from build123d import *

# Parameters (mm, degrees)
F0_W     = 70
F0_H     = 60
F1_DEPTH = 20
F2_R     = 7
F3_T     = -3
F4_R     = 4.7885075057
F4_R_2   = 3.7026235456
F5_DEPTH = 1


with BuildPart() as f1:
    # F0 (on Front) → F1 (new body)
    with BuildSketch(Plane.XZ):
        Rectangle(F0_W, F0_H)
    extrude(amount=F1_DEPTH)

    # F2
    f2_edges = [f1.edges().sort_by_distance(p)[0] for p in [
        (35, -10, -30),
        (-35, -10, -30),
        (35, -10, 30),
        (-35, -10, 30),
    ]]
    fillet(f2_edges, radius=F2_R)

    # F3
    f3_openings = [f1.faces().sort_by_distance(p)[0] for p in [
        (0, 0, 0),
    ]]
    offset(amount=F3_T, openings=f3_openings)

    # F4 (on face) → F5 (cut)
    with BuildSketch(Plane.XZ.offset(20)):
        with BuildLine():
            ThreePointArc((5.9756954083, -21.3208798361), (7.5060376285, -18.8306109679), (8.0398977368, -15.9568712908))
            ThreePointArc((8.0398977368, -15.9568712908), (7.9036150749, -14.4863732956), (7.4994094473, -13.0659666184))
            Line((7.4994094473, -13.0659666184), (6.1305917901, -14.4159711191))
            ThreePointArc((6.1305917901, -14.4159711191), (6.2842749217, -15.2041179655), (6.3357852508, -16.0054547502))
            ThreePointArc((6.3357852508, -16.0054547502), (-5.5540754685, -18.7377869694), (3.9501702088, -11.0890131208))
            Line((3.9501702088, -11.0890131208), (5.196705387, -9.840010404))
            ThreePointArc((5.196705387, -9.840010404), (-7.9557042611, -15.6118703464), (4.6505361801, -22.4953976897))
            ThreePointArc((4.6505361801, -22.4953976897), (5.3457061154, -21.9449090553), (5.9756954083, -21.3208798361))
        make_face()
        with BuildLine():
            Line((0.0383761635, -19.0379637991), (5.7637177193, -13.3913118671))
            ThreePointArc((5.7637177193, -13.3913118671), (5.3063853455, -12.5665425426), (4.7303228045, -11.8198503118))
            Line((4.7303228045, -11.8198503118), (0.0383761635, -16.4483864674))
            Line((0.0383761635, -16.4483864674), (-2.3087403007, -14.0691147408))
            ThreePointArc((-2.3087403007, -14.0691147408), (-3.6156147651, -14.0808212911), (-3.5627264086, -15.386677612))
            Line((-3.5627264086, -15.386677612), (0.0383761635, -19.0379637991))
        make_face()
        with BuildLine():
            Line((5.7637177193, -13.3913118671), (7.0574382874, -12.1153723141))
            ThreePointArc((7.0574382874, -12.1153723141), (6.5608204438, -11.3219960932), (5.9749529426, -10.5920410388))
            Line((5.9749529426, -10.5920410388), (4.7303228045, -11.8198503118))
            ThreePointArc((4.7303228045, -11.8198503118), (5.3063853455, -12.5665425426), (5.7637177193, -13.3913118671))
        make_face()
        with BuildLine():
            ThreePointArc((5.9749529426, -10.5920410388), (6.5608204438, -11.3219960932), (7.0574382874, -12.1153723141))
            Line((7.0574382874, -12.1153723141), (10.3152280376, -8.9023579275))
            ThreePointArc((10.3152280376, -8.9023579275), (10.3242561937, -7.5976353085), (9.0195335747, -7.5886071525))
            Line((9.0195335747, -7.5886071525), (5.9749529426, -10.5920410388))
        make_face()
        with BuildLine():
            Line((-25.463836038, 14.5788419077), (-29.0132504877, 14.5788419077))
            Line((-29.0132504877, 14.5788419077), (-29.0132504877, 5.0767470373))
            Line((-29.0132504877, 5.0767470373), (-24.9086179807, 5.0767470373))
            ThreePointArc((-24.9086179807, 5.0767470373), (-22.7022924412, 7.5970867281), (-24.2285804935, 10.5787690258))
            ThreePointArc((-24.2285804935, 10.5787690258), (-23.7062839611, 12.9308235072), (-25.463836038, 14.5788419077))
        make_face()
        with BuildLine():
            Line((-27.9734000776, 10.8749483858), (-27.9734000776, 13.5894283968))
            Line((-27.9734000776, 13.5894283968), (-25.6162118383, 13.5894283968))
            ThreePointArc((-25.6162118383, 13.5894283968), (-24.6244842165, 12.2231458353), (-25.6406610471, 10.8749483858))
            Line((-25.6406610471, 10.8749483858), (-27.9734000776, 10.8749483858))
        make_face(mode=Mode.SUBTRACT)
        with BuildLine():
            Line((-27.9640843056, 9.8444300713), (-25.0821946304, 9.8444300713))
            ThreePointArc((-25.0821946304, 9.8444300713), (-23.7118512956, 8.0211258), (-25.0821946304, 6.1978215287))
            Line((-25.0821946304, 6.1978215287), (-27.9640843056, 6.188870993))
            Line((-27.9640843056, 6.188870993), (-27.9640843056, 9.8444300713))
        make_face(mode=Mode.SUBTRACT)
        with BuildLine():
            ThreePointArc((-19.3660976033, 14.2887552617), (-19.8752782584, 14.8065162395), (-20.40147499, 14.30605808))
            Line((-20.40147499, 14.30605808), (-20.40147499, 5.4078511567))
            ThreePointArc((-20.40147499, 5.4078511567), (-19.884282799, 5.1317819915), (-19.3660976033, 5.405982738))
            Line((-19.3660976033, 5.405982738), (-19.3660976033, 14.2887552617))
        make_face()
        with Locations((-12.3437182241, 9.891309084)):
            Circle(F4_R)
        with Locations((-12.3052396193, 9.8635797819)):
            Circle(F4_R_2, mode=Mode.SUBTRACT)
        Polygon((0.060495557, 14.6499899539), (-6.2339946938, 14.6499899539), (-6.2279876776, 13.6288518889), (-3.5691043968, 13.6288518889), (-3.5691043968, 5.3356449452), (-2.5498712742, 5.3356449452), (-2.5498712742, 13.6288518889), (0.060495557, 13.6288518889), align=None)
        with BuildLine():
            ThreePointArc((0.060495557, 13.6288518889), (0.5710645895, 14.1394209214), (0.060495557, 14.6499899539))
            Line((0.060495557, 14.6499899539), (0.060495557, 13.6288518889))
        make_face()
        with BuildLine():
            Line((-6.2279876776, 13.6288518889), (-6.2339946938, 14.6499899539))
            ThreePointArc((-6.2339946938, 14.6499899539), (-6.7385655444, 14.13643503), (-6.2279876776, 13.6288518889))
        make_face()
        with BuildLine():
            Line((5.68894728, 14.6499899539), (2.3992179348, 14.6499899539))
            Line((2.3992179348, 14.6499899539), (2.3992179348, 5.4546332436))
            ThreePointArc((2.3992179348, 5.4546332436), (2.9464930191, 5.1446017563), (3.4937681035, 5.4546332436))
            Line((3.4937681035, 5.4546332436), (3.4937681035, 8.8353623544))
            Line((3.4937681035, 8.8353623544), (5.4684750956, 8.8353623544))
            Line((5.4684750956, 8.8353623544), (7.6643496496, 5.2591634276))
            ThreePointArc((7.6643496496, 5.2591634276), (8.3467179976, 5.2108037756), (8.6122971182, 5.8412266091))
            Line((8.6122971182, 5.8412266091), (6.5826675849, 9.1466790748))
            ThreePointArc((6.5826675849, 9.1466790748), (8.1293427353, 12.2220783511), (5.68894728, 14.6499899539))
        make_face()
        with BuildLine():
            ThreePointArc((5.68894728, 13.6319459919), (7.0831009819, 11.7494924749), (5.5949211536, 9.9404549997))
            Line((5.5949211536, 9.9404549997), (3.3746365671, 9.9404549997))
            Line((3.3746365671, 9.9404549997), (3.3746365671, 13.6319459919))
            Line((3.3746365671, 13.6319459919), (5.68894728, 13.6319459919))
        make_face(mode=Mode.SUBTRACT)
        with BuildLine():
            ThreePointArc((14.7096056189, 14.4168665306), (14.3134062852, 14.6801129854), (13.9264534318, 14.4034541752))
            Line((13.9264534318, 14.4034541752), (10.6487381189, 5.9825136642))
            ThreePointArc((10.6487381189, 5.9825136642), (10.9675570687, 5.2573357806), (11.6927349523, 5.5761547304))
            Line((11.6927349523, 5.5761547304), (12.7655428348, 8.3323585177))
            Line((12.7655428348, 8.3323585177), (16.0099739306, 8.3323585177))
            Line((16.0099739306, 8.3323585177), (17.1330149852, 5.5268825081))
            ThreePointArc((17.1330149852, 5.5268825081), (17.8181026735, 5.2334854183), (18.1114997633, 5.9185731066))
            Line((18.1114997633, 5.9185731066), (14.7096056189, 14.4168665306))
        make_face()
        Polygon((13.1405137187, 9.48174586), (14.4126430381, 12.6535973069), (15.6418385154, 9.48174586), align=None, mode=Mode.SUBTRACT)
        with BuildLine():
            ThreePointArc((27.6586074546, 10.8364686124), (27.7543057203, 10.3589358747), (27.7863908123, 9.8729665129))
            ThreePointArc((27.7863908123, 9.8729665129), (20.7773970324, 8.2330148821), (26.3312045231, 12.8123879303))
            Line((26.3312045231, 12.8123879303), (27.0641849046, 13.6325057938))
            ThreePointArc((27.0641849046, 13.6325057938), (19.2418374627, 10.0479724553), (26.81568619, 5.9644918061))
            ThreePointArc((26.81568619, 5.9644918061), (27.2455005085, 6.3059753785), (27.6335724386, 6.6942427552))
            ThreePointArc((27.6335724386, 6.6942427552), (28.5370532464, 8.1811527366), (28.851969289, 9.8922946796))
            ThreePointArc((28.851969289, 9.8922946796), (28.7631907726, 10.8118138528), (28.5001349107, 11.6973638223))
            Line((28.5001349107, 11.6973638223), (27.6586074546, 10.8364686124))
        make_face()
        with BuildLine():
            Line((24.0681641205, 8.0956717688), (27.4159314963, 11.4858697823))
            ThreePointArc((27.4159314963, 11.4858697823), (27.1680184196, 11.9196861576), (26.8638629672, 12.316103869))
            Line((26.8638629672, 12.316103869), (24.0900374708, 9.5071220515))
            Line((24.0900374708, 9.5071220515), (22.775273925, 10.8054304358))
            ThreePointArc((22.775273925, 10.8054304358), (22.0626570945, 10.8039400184), (22.0641475119, 10.0913231879))
            Line((22.0641475119, 10.0913231879), (24.0681641205, 8.0956717688))
        make_face()
        with BuildLine():
            ThreePointArc((27.6335724386, 6.6942427552), (27.2455005085, 6.3059753785), (26.81568619, 5.9644918061))
            Line((26.81568619, 5.9644918061), (28.4407067429, 4.1904454021))
            ThreePointArc((28.4407067429, 4.1904454021), (29.214969102, 4.1564992903), (29.2489152138, 4.9307616493))
            Line((29.2489152138, 4.9307616493), (27.6335724386, 6.6942427552))
        make_face()
        with BuildLine():
            ThreePointArc((27.6311249444, 13.0930903614), (27.9416464389, 12.7068871234), (28.2107508353, 12.2907629071))
            Line((28.2107508353, 12.2907629071), (29.647856175, 13.7460825638))
            ThreePointArc((29.647856175, 13.7460825638), (29.6435095117, 14.4363306609), (28.9532614146, 14.4319839976))
            Line((28.9532614146, 14.4319839976), (27.6311249444, 13.0930903614))
        make_face()
        with BuildLine():
            ThreePointArc((26.8638629672, 12.316103869), (27.1680184196, 11.9196861576), (27.4159314963, 11.4858697823))
            Line((27.4159314963, 11.4858697823), (28.2107508353, 12.2907629071))
            ThreePointArc((28.2107508353, 12.2907629071), (27.9416464389, 12.7068871234), (27.6311249444, 13.0930903614))
            Line((27.6311249444, 13.0930903614), (26.8638629672, 12.316103869))
        make_face()
    extrude(amount=-F5_DEPTH, mode=Mode.SUBTRACT)


solid = f1.part
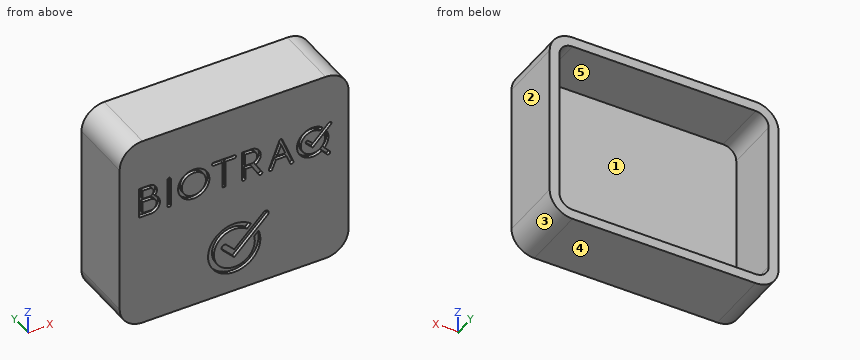
Source: CAD feature listing. Evaluate the final solid. Frame: model axes, mm. Face numbers are marked on the shaded views. A direction names the side the tool comes from. Round coordinates to 2 decimals unless told otherwise and drop trailing zeros. Loops run counter-clockwise (first coordinate to the right, second up) from the corner with the lowest first, then second, coordinate; pieces in that order, holes last.
Q1. Ray query, line 1 (X direction, y = -6.5, z = 17); line 2 (Z direction, x = -8, y = -10.5); line 3 (Y direction, x = -15, z = -20). Return the intervals inside material, ascending.
Q2. First-contact query: P1, Ø8.5, axis at x = -12.34, z = 9.89, coming from the +Y side. Flat tip, straight axial feed; report the tip coordinate or a pass-through.
Q3. Section A-A, the plane y = -13.75. Return loops of the section in (x, z).
Q4. Section D-D, the plane x = -12.5. Return loops of the section in (y, z).
Q5. Access query for the marked faces 1 and 2. Directions: +Z, -Z, +X, -X, +Y, -Y. A direction counts if a zero-diameter tool reaches every point of the face in a straight line with its end or side. Return the directions, or none.
Q6. Mould query, pull axis X, two halves, no side actions, for the marked faces 3, 4 and 5. Classes: pulls with the +X half, pulls with the -X half, needs draft (parallel to the pull), parting line crosses it, or undercut.
Q7. Section B-B, the plane z = 18. Return loops of the section in (x, y), plus the area to 3 significant figures.
Q8. Section C-C, the plane x = -26.5. Return loops of the section in (y, z), plus the area to 3 significant figures.
Solutions:
1. line 1: x = -35 to -32, 32 to 35
1. line 2: z = -30 to -27, 27 to 30
1. line 3: y = -20 to -17
2. P1: stops at y = -17
3. outline: (-35, -23) arc R7 ccw to (-28, -30) - (28, -30) arc R7 ccw to (35, -23) - (35, 23) arc R7 ccw to (28, 30) - (-28, 30) arc R7 ccw to (-35, 23) - close; hole (-32, -23) arc R4 ccw to (-28, -27) - (28, -27) arc R4 ccw to (32, -23) - (32, 23) arc R4 ccw to (28, 27) - (-28, 27) arc R4 ccw to (-32, 23) - close
4. outline: (-20, -30) - (0, -30) - (0, -27) - (-17, -27) - (-17, 27) - (0, 27) - (0, 30) - (-20, 30) - (-20, 14.68) - (-19, 14.68) - (-19, 13.56) - (-20, 13.56) - (-20, 6.17) - (-19, 6.17) - (-19, 5.11) - (-20, 5.11) - close
5. face 1: +Y
5. face 2: +Z, -Z, +X, +Y, -Y
6. face 3: pulls with the +X half
6. face 4: needs draft
6. face 5: undercut
7. outline: (-35, -20) - (35, -20) - (35, 0) - (32, 0) - (32, -17) - (-32, -17) - (-32, 0) - (-35, 0) - close
7. area: 312 mm2
8. outline: (-20, -30) - (0, -30) - (0, -27) - (-17, -27) - (-17, 27) - (0, 27) - (0, 30) - (-20, 30) - (-20, 14.58) - (-19, 14.58) - (-19, 13.59) - (-20, 13.59) - (-20, 10.87) - (-19, 10.87) - (-19, 9.84) - (-20, 9.84) - (-20, 6.19) - (-19, 6.19) - (-19, 5.08) - (-20, 5.08) - close
8. area: 279 mm2
